The model under review builds one solid part; all positions refer to its coordinate system, in mm. Face numbers are marked on the shaded views. Round coordinates to 2 decimals unless told otherwise and drop trailing zeros. Write each loop counter-clockwise with the first axis right and the second up, starting at its lowest first coordinate (ties: lowest second). Pieces come first, ordered by that corner, then holes.
Item 1: Draft analysis for pull direction Y (two halves, no side actions). For the marked faces 1, 2, 3 and 4, state which applies: +Y half, -Y half, draft (parallel to the pull), parting line (faces both ways), or undercut.
Item 2: Clearance check with a flat-ended pin moving along its axis: pin 1 Ø9 at (y, z) = (0, 26) entering from -X. State where the tip first meets the part, or that it passes through.
Item 3: Add section A-A (z = 26). Give the boundary of the cut face in (x, y), plus the area to 3 significant figures.
Item 4: Add section B-B (y = 0). Give the boundary of the cut face in (x, z), plus the area to 3 significant figures.
Item 5: To check wall thickness, follow L1, parallel to Z at x = -18, y = 0. State the ranges of the line that lie inside material, in increasing order.
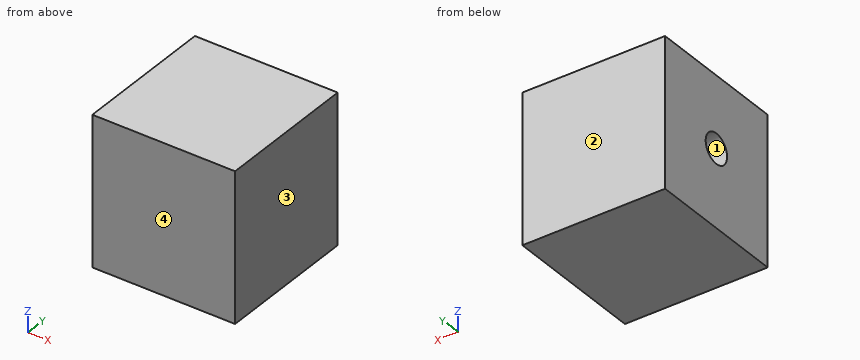
```python
from build123d import *

# Parameters (mm, degrees)
CROQUIS1_W              = 48
CROQUIS1_H              = 48
SALIENTE_EXTRUIR1_DEPTH = 50
CROQUIS3_R              = 5
CORTAR_EXTRUIR2_DEPTH   = 10


with BuildPart() as part:
    # Croquis1 → Saliente-Extruir1 (new body)
    with BuildSketch(Plane.XY):
        Rectangle(CROQUIS1_W, CROQUIS1_H)
    extrude(amount=SALIENTE_EXTRUIR1_DEPTH)

    # Croquis3 → Cortar-Extruir2 (cut)
    with BuildSketch(Plane.ZY.offset(24)):
        with Locations(Location((26, 0, 0), (0, 0, 270))):
            Circle(CROQUIS3_R)
    extrude(amount=-CORTAR_EXTRUIR2_DEPTH, mode=Mode.SUBTRACT)


solid = part.part
```
Numbers:
1. face 1: undercut
1. face 2: +Y half
1. face 3: draft
1. face 4: -Y half
2. pin 1: stops at x = -14
3. outline: (-24, -24) - (24, -24) - (24, 24) - (-24, 24) - (-24, 5) - (-14, 5) - (-14, -5) - (-24, -5) - close
3. area: 2,200 mm2
4. outline: (-24, 0) - (24, 0) - (24, 50) - (-24, 50) - (-24, 31) - (-14, 31) - (-14, 21) - (-24, 21) - close
4. area: 2,300 mm2
5. L1: z = 0 to 21, 31 to 50
